Here's how the part is built. I have some questions about the finished solid (model axes, mm). Coordinates: 2 decimals unless noted, no trailing zeros. Loops run counter-clockwise (first coordinate to the right, second up) from the corner with the lowest first, then second, coordinate; pieces in that order, holes last. Notation, with made-up numbers: M -13,-37.75 L -7,-37.75 A32 ccw -7,-0.75 Z; hole C 36.25,54 d7. An arc over 180 degrees is marked long. Use CSV: the item, a comma, the result in double quotes. Start each with the question number.
Q1. Please list where these lines run through material, in increasing order: probe 1 along Y at (x, z) = (0, 72); probe 2 along X at (y, z) = (-2.5, -41) (3 decimals); probe 3 along X at (y, z) = (2.75, 128.5). Write a range as [from, to].
Q2. If we section it at D-D (x = -8): Please give me the cut outline in (y, z) (3 decimals).
Q3. If we section it at A-A (z = 55): Please give me the cut outline in (x, y) (3 decimals), and give its area (3 significant figures).
Q4. If we section it at C-C (z = -72): Please give me the cut outline in (x, y) (3 decimals), and give its area (3 significant figures).
Q5. If we section it at B-B (y = 0): Please give me the cut outline in (x, z) (3 decimals).
Q6. For pin 1 Ø2 at (x, y) = (-32.5, 4) entering from -Z; pin 2 Ø12 at (x, z) = (-31.5, 20) entering from -Y (3 decimals); pin 3 Ø5 at (y, z) = (0.5, 128.5) entering from +X; pin 4 Ø21 at (x, z) = (-18.5, 76) entering from +Y, each with a flat end and sliding along its axis, tell me the tip position at first contact or that it passes through.
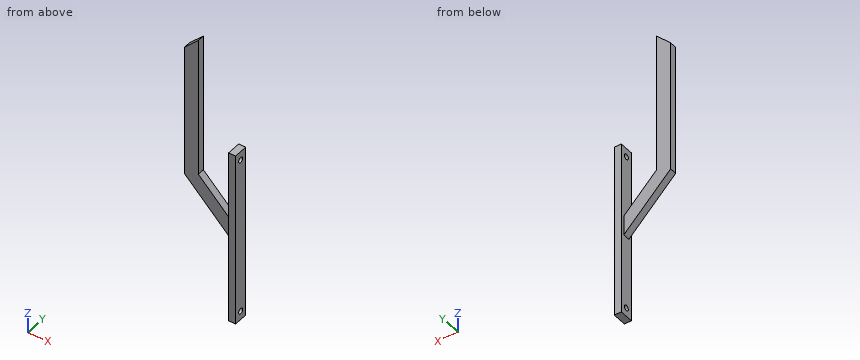
from build123d import *

# Parameters (mm, degrees)
BOSS_EXTRUDE1_DEPTH      = 80
BOSS_EXTRUDE1_DEPTH_BACK = 80
SKETCH2_W                = 6.35
SKETCH2_H                = 12.7
SKETCH4_R                = 2.5
CUT_EXTRUDE1_DEPTH       = 81.502453379
BOSS_EXTRUDE2_DEPTH      = 3.175
BOSS_EXTRUDE2_DEPTH_BACK = 3.175


with BuildPart() as part:
    # Sketch2 → Boss-Extrude1 (new, two sides: drawn at the far end of the back side and taken through both)
    with BuildSketch(Plane.XY.offset(-BOSS_EXTRUDE1_DEPTH_BACK)):
        Rectangle(SKETCH2_W, SKETCH2_H)
    extrude(amount=BOSS_EXTRUDE1_DEPTH + BOSS_EXTRUDE1_DEPTH_BACK)

    # Sketch4 → Cut-Extrude1 (cut, through all)
    with BuildSketch(Plane(origin=(3.175, 0, 0), x_dir=(0, 0, -1), z_dir=(1, 0, 0))):
        with Locations((-72, 0)):
            Circle(SKETCH4_R)
        with Locations(Location((72, 0, 0), (0, 0, 180))):
            Circle(SKETCH4_R)
    extrude(amount=-CUT_EXTRUDE1_DEPTH, mode=Mode.SUBTRACT)

    # Sketch5 → Boss-Extrude2 (add, two sides: drawn at the far end of the back side and taken through both)
    with BuildSketch(Plane(origin=(0, 0, 0), x_dir=(0, 0, -1), z_dir=(0, 1, 0)).offset(-BOSS_EXTRUDE2_DEPTH_BACK)):
        Polygon((4.490128061, 3.175), (-37.936278811, 45.601406871), (-157.936278811, 45.601406871), (-170.636278811, 32.901406871), (-43.196791053, 32.901406871), (-7.120384182, -3.175), (-1.859871939, -3.175), align=None)
    extrude(amount=BOSS_EXTRUDE2_DEPTH + BOSS_EXTRUDE2_DEPTH_BACK)


solid = part.part
Results below:
1,probe 1,"[-6.35, -2.5], [2.5, 6.35]"
1,probe 2,"[-3.175, 3.175]"
1,probe 3,"[-45.6, -32.9]"
2,outline,"M -3.175,0.335 L 3.175,0.335 L 3.175,18.295 L -3.175,18.295 Z"
3,outline,"M -45.601,-3.175 L -32.901,-3.175 L -32.901,3.175 L -45.601,3.175 Z; M -3.175,-6.35 L 3.175,-6.35 L 3.175,6.35 L -3.175,6.35 Z"
3,area,"161 mm^2"
4,outline,"M -3.175,-6.35 L 3.175,-6.35 L 3.175,-2.5 L -3.175,-2.5 Z; M -3.175,2.5 L 3.175,2.5 L 3.175,6.35 L -3.175,6.35 Z"
4,area,"48.9 mm^2"
5,outline,"M -45.601,37.936 L -3.175,-4.49 L -3.175,-69.5 L 3.175,-69.5 L 3.175,69.5 L -3.175,69.5 L -3.175,13.47 L -32.901,43.197 L -32.901,170.636 L -45.601,157.936 Z; M -3.175,-80 L 3.175,-80 L 3.175,-74.5 L -3.175,-74.5 Z; M -3.175,74.5 L 3.175,74.5 L 3.175,80 L -3.175,80 Z"
6,pin 1,"z = 24.27"
6,pin 2,"y = -3.175"
6,pin 3,"x = -32.9"
6,pin 4,"through"
